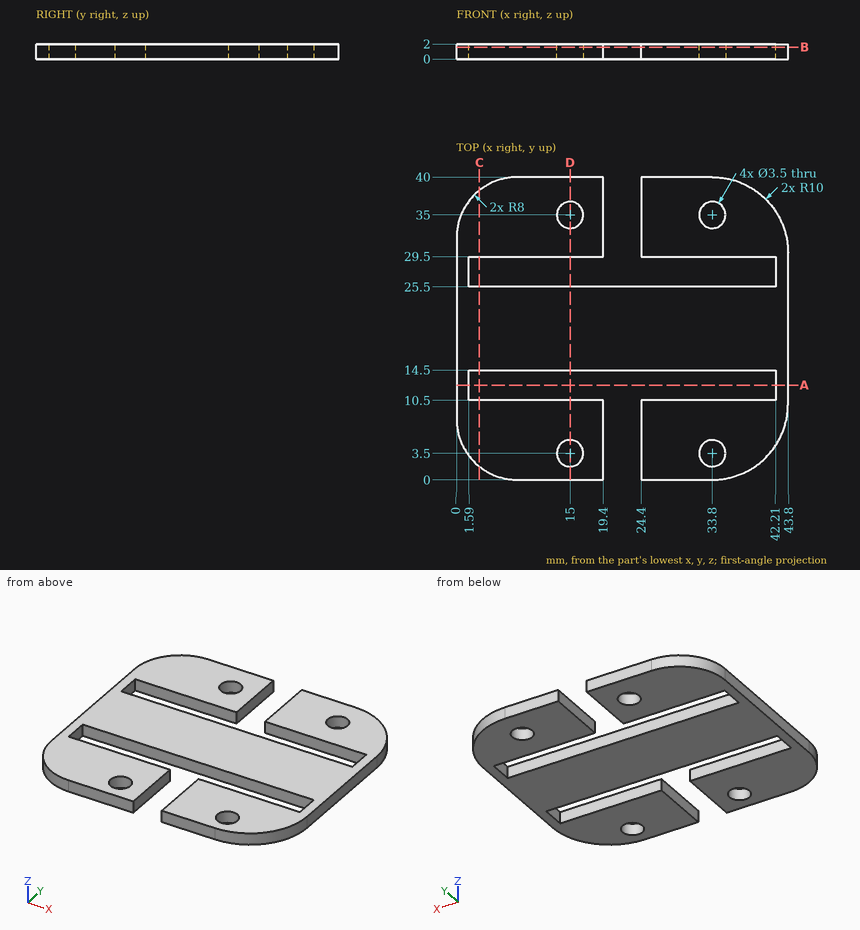
Can you work these out from the drawing? Everything is in mm from the part's minimum corner. Coordinates: 2 decimals unless noted, no trailing zeros. Loops run counter-clockwise (first coordinate to the right, second up) from the corner with the lowest first, then second, coordinate; pieces in that order, holes last.
1) Imagine slicing it at C-C on x = 3. List the corners of the cut face in (y, z) for me (3 decimals).
2) Imagine slicing it at D-D on x = 15. List the corners of the cut face in (y, z) for me, plus the area to 3 significant figures.
3) Imagine slicing it at A-A on y = 12.5. List the corners of the cut face in (x, z) for me, plus the area to 3 significant figures.
4) I need wall thicknesses on probe 1 along Y at (x, z) = (33.8, 1.6); probe 2 along Y at (x, z) = (31, 1.9); probe 3 along X at (y, z) = (13.5, 0.75). Which ranges of each line are inside material? Lowest first, please.
5) For pin 1 (0.6 mm diameter, centred on y = 33, z = 1.5, fed in from +X); pin 2 (0.6 mm diameter, centred on y = 34, z = 1, fed in from -X); pin 3 (0.6 mm diameter, centred on y = 4.5, z = 1.5, fed in from -X), each with a flat end and sliding along its axis, tell me the tip position at first contact or that it passes through.
6) Imagine slicing it at B-B on z = 1.6. List the corners of the cut face in (x, y) for me, plus the area to 3 significant figures.
Completed:
1. outline: (1.755, 0) - (10.5, 0) - (10.5, 2) - (1.755, 2) - close; (14.5, 0) - (25.5, 0) - (25.5, 2) - (14.5, 2) - close; (29.5, 0) - (38.245, 0) - (38.245, 2) - (29.5, 2) - close
2. outline: (0, 0) - (1.75, 0) - (1.75, 2) - (0, 2) - close; (5.25, 0) - (10.5, 0) - (10.5, 2) - (5.25, 2) - close; (14.5, 0) - (25.5, 0) - (25.5, 2) - (14.5, 2) - close; (29.5, 0) - (33.25, 0) - (33.25, 2) - (29.5, 2) - close; (36.75, 0) - (40, 0) - (40, 2) - (36.75, 2) - close
2. area: 50.0 mm2
3. outline: (0, 0) - (1.59, 0) - (1.59, 2) - (0, 2) - close; (42.21, 0) - (43.8, 0) - (43.8, 2) - (42.21, 2) - close
3. area: 6.36 mm2
4. probe 1: y = 0 to 1.75, 5.25 to 10.5, 14.5 to 25.5, 29.5 to 33.25, 36.75 to 40
4. probe 2: y = 0 to 10.5, 14.5 to 25.5, 29.5 to 40
4. probe 3: x = 0 to 1.59, 42.21 to 43.8
5. pin 1: stops at x = 43.43
5. pin 2: stops at x = 0.18
5. pin 3: stops at x = 0.67
6. outline: (0, 8) arc R8 ccw to (8, 0) - (19.4, 0) - (19.4, 10.5) - (1.59, 10.5) - (1.59, 14.5) - (42.21, 14.5) - (42.21, 10.5) - (24.4, 10.5) - (24.4, 0) - (33.8, 0) arc R10 ccw to (43.8, 10) - (43.8, 30) arc R10 ccw to (33.8, 40) - (24.4, 40) - (24.4, 29.5) - (42.21, 29.5) - (42.21, 25.5) - (1.59, 25.5) - (1.59, 29.5) - (19.4, 29.5) - (19.4, 40) - (8, 40) arc R8 ccw to (0, 32) - close; hole circle Ø3.5 at (15, 3.5); hole circle Ø3.5 at (15, 35); hole circle Ø3.5 at (33.8, 3.5); hole circle Ø3.5 at (33.8, 35)
6. area: 1,210 mm2
